```python
from build123d import *

# Parameters (mm, degrees)
SKETCH1_W           = 16.5
SKETCH1_H           = 16.5
SKETCH1_R           = 1.375
BOSS_EXTRUDE1_DEPTH = 2.5
SKETCH2_R           = 4.75
SKETCH2_R_2         = 1.375
BOSS_EXTRUDE2_DEPTH = 70


with BuildPart() as part:
    # Sketch1 → Boss-Extrude1 (new body)
    with BuildSketch(Plane(origin=(0, 0, 0), x_dir=(1, 0, 0), z_dir=(0, 1, 0))):
        with Locations((0.455521472, -1.417177914)):
            Rectangle(SKETCH1_W, SKETCH1_H)
        with Locations((0.455521472, -1.417177914)):
            Circle(SKETCH1_R, mode=Mode.SUBTRACT)
    extrude(amount=BOSS_EXTRUDE1_DEPTH)

    # Sketch2 → Boss-Extrude2 (add)
    with BuildSketch(Plane(origin=(0, 2.5, 0), x_dir=(1, 0, 0), z_dir=(0, 1, 0))):
        with Locations((0.455521472, -1.417177914)):
            Circle(SKETCH2_R)
        with Locations((0.455521472, -1.417177914)):
            Circle(SKETCH2_R_2, mode=Mode.SUBTRACT)
    extrude(amount=BOSS_EXTRUDE2_DEPTH)


solid = part.part
```
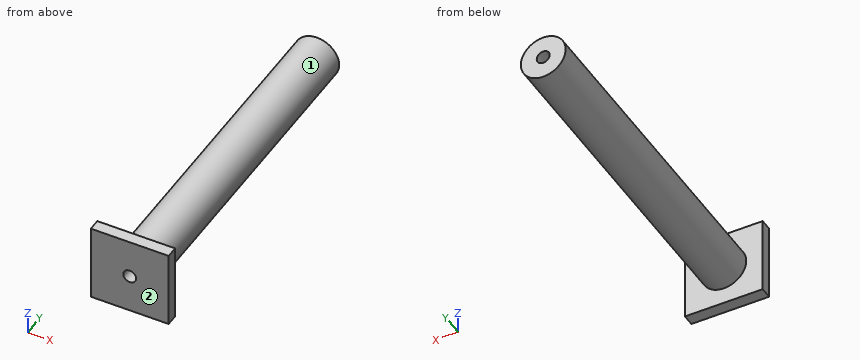
The listing builds one solid part. Answer for the finished solid, in the listing's coordinates (mm). Face numbers are marked on the shaded views. A direction names the side the tool comes from. Round coordinates to 2 decimals unless told otherwise and drop trailing zeros. Write each loop counter-clockwise with the first axis right and the second up, starting at its lowest first coordinate (ties: lowest second). Pieces come first, ordered by that corner, then holes. Notation, with made-up numbers: (71.5, 0.5) -> (76.5, 0.5) arc R25 ccw to (76.5, 20.5) -> close; hole circle Ø4 at (67.25, 80). An arc over 180 degrees is marked (long way). Use CSV: the item, a comma, the result in double quotes. Start each with the question number.
(1) Each of these flat-tipped pins is pushed along its axis until it touches: pin 1 (6 mm diameter, centred on x = 6, y = 15, fed in from -Z); pin 2 (1 mm diameter, centred on x = 2, y = 28, fed in from -Z); pin 3 (8 mm diameter, centred on x = -1, y = 47.5, fed in from +Z). Where does it stop, or does it pass through?
(2) Section B-B on z = 3.75 is taken. Give the vertices of the cut face in (x, y).
(3) Section A-A on x = 0 is taken. Give the vertices of the cut face in (y, z).
(4) Section C-C on y = 54 is taken. Give the vertices of the cut face in (x, z) (3 decimals), then the cut area to 3 significant figures.
(5) Section D-D on x = 2.75 is taken. Give the vertices of the cut face in (y, z).
(6) Which of the six approach directions +Z, -Z, +X, -X, +Y, -Y give full straight-line access (tool end or side, diameter ignored) to the marked faces 1 and 2?
(7) Consider L1, parallel to Y at x = 5.75, z = -2.5; L2, parallel to Z at x = 0.5, y = 54; L3, parallel to X at y = 44.5, z = 1.25. Determine where each line is inside the solid, lowest interval first. Write a range as from..to.
A:
1,pin 1,"stops at z = -2.59"
1,pin 2,"stops at z = -3.22"
1,pin 3,"stops at z = 6.17"
2,outline,"(-7.79, 0) -> (8.71, 0) -> (8.71, 2.5) -> (4.59, 2.5) -> (4.59, 72.5) -> (-3.68, 72.5) -> (-3.68, 2.5) -> (-7.79, 2.5) -> close"
3,outline,"(0, -6.83) -> (2.5, -6.83) -> (2.5, -3.31) -> (72.5, -3.31) -> (72.5, 0.12) -> (0, 0.12) -> close; (0, 2.71) -> (72.5, 2.71) -> (72.5, 6.15) -> (2.5, 6.15) -> (2.5, 9.67) -> (0, 9.67) -> close"
4,outline,"circle Ø9.5 at (0.456, 1.417); hole circle Ø2.75 at (0.456, 1.417)"
4,area,"64.9 mm²"
5,outline,"(0, -6.83) -> (2.5, -6.83) -> (2.5, -2.74) -> (72.5, -2.74) -> (72.5, 5.58) -> (2.5, 5.58) -> (2.5, 9.67) -> (0, 9.67) -> close"
6,face 1,"+Y"
6,face 2,"+Z, -Z, +X, -X, -Y"
7,L1,"y = 0..2.5"
7,L2,"z = -3.33..0.04, 2.79..6.17"
7,L3,"x = -4.29..-0.91, 1.82..5.2"
